Could you check a few things on this drawing? It's one solid part, dimensions in mm from its lowest x, y, z. Give positions to 0.01 mm unless a question says otherwise; leave off trailing zeros. Order: outer loops, then holes, each group sorted by start corner. A loop starts at its lowest first (then second) coordinate and runs counter-clockwise, first axis right, second up.
Item 1: I want a section at B-B, the plane y = 6.5. Write out the boundary of the cut face in (x, z), then the cut area to 3 significant figures.
Item 2: I want a section at C-C, the plane x = 24. Write out the boundary of the cut face in (y, z), then the cut area to 3 significant figures.
Item 3: I want a section at D-D, the plane x = 17. Write out the boundary of the cut face in (y, z).
Item 4: I want a section at A-A, the plane z = 7.5. Write out the boundary of the cut face in (x, y).
Item 5: I'm going to push flat-ended pins straight in: pin 1 Ø2 at (y, z) = (18, 61) entering from -X; pin 2 Ø3 at (x, y) = (25, 44.5) entering from -Z; pin 3 Ø1.5 at (x, y) = (32.5, 42.5) entering from +Z; pin 4 Ø6 at (x, y) = (16, 33) entering from +Z. Where does each tip first touch, or does it pass through?
Item 6: If I drill on line 1 along X through (y, z) = (40.5, 16.5); line 2 along Z through (x, y) = (29.5, 16.5); line 3 along X through (y, z) = (9, 67.5) (1 decimal), over which ranges is the centre line in solid material (lowest first)?
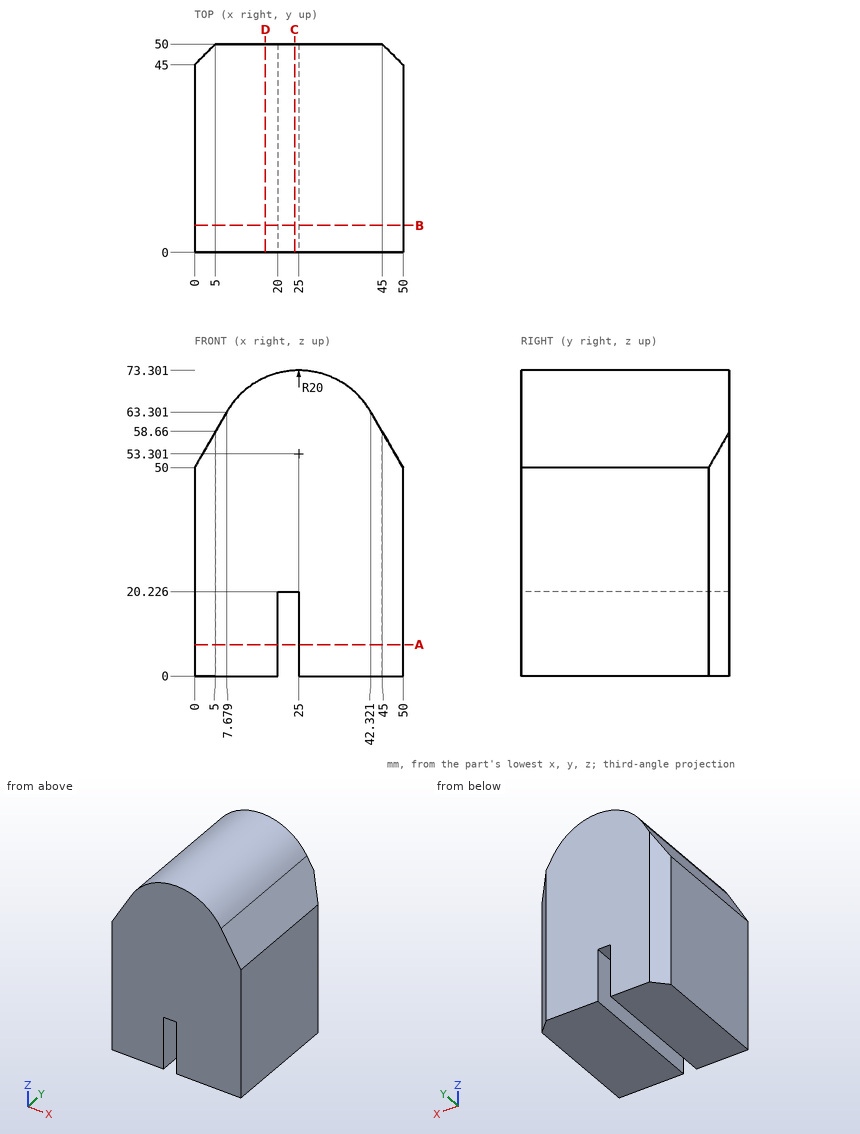
Results list:
1. outline: (0, 0) - (20, 0) - (20, 20.23) - (25, 20.23) - (25, 0) - (50, 0) - (50, 50) - (42.32, 63.3) arc R20 ccw to (7.68, 63.3) - (0, 50) - close
1. area: 3,210 mm2
2. outline: (0, 20.23) - (50, 20.23) - (50, 73.28) - (0, 73.28) - close
2. area: 2,650 mm2
3. outline: (0, 0) - (50, 0) - (50, 71.63) - (0, 71.63) - close
4. outline: (0, 0) - (20, 0) - (20, 50) - (5, 50) - (0, 45) - close; (25, 0) - (50, 0) - (50, 45) - (45, 50) - (25, 50) - close
5. pin 1: stops at x = 5.77
5. pin 2: stops at z = 0
5. pin 3: stops at z = 72.13
5. pin 4: stops at z = 72.38
6. line 1: x = 0 to 20, 25 to 50
6. line 2: z = 0 to 72.79
6. line 3: x = 10.9 to 39.1
